Part model, mm, in its own coordinate system. Round coordinates to 2 decimals unless told otherwise and drop trailing zeros. Write each loop counter-clockwise with the first axis right and the second up, starting at its lowest first coordinate (ties: lowest second). Pieces come first, ordered by that corner, then holes. Notation, with made-up numbers: (5, 89) -> (57, 89) arc R25 ccw to (57, 124) -> close; hole circle Ø9 at (32, 1). An arc over 180 degrees is marked (long way). Return JSON: item names as keys, results as strings. Group by question number.
```python
from build123d import *

# Parameters (mm, degrees)
SKETCH1_W            = 44
SKETCH1_H            = 45.6
BOSS_EXTRUDE1_DEPTH  = 18
FILLET1_R            = 3
M4_CLEARANCE_HOLE1_D = 4.5


with BuildPart() as part:
    # Sketch1 → Boss-Extrude1 (new body)
    with BuildSketch(Plane(origin=(0, 0, 0), x_dir=(1, 0, 0), z_dir=(0, 1, 0))):
        Rectangle(SKETCH1_W, SKETCH1_H)
    extrude(amount=BOSS_EXTRUDE1_DEPTH)

    # Fillet1
    fillet1_edges = [part.edges().sort_by_distance(p)[0] for p in [
        (22, 9, 22.8),
        (-22, 9, 22.8),
        (-22, 9, -22.8),
        (22, 9, -22.8),
    ]]
    fillet(fillet1_edges, radius=FILLET1_R)

    # M4 Clearance Hole1 (through all)
    with Locations(Plane(origin=(0, 18, 0), x_dir=(1, 0, 0), z_dir=(0, 1, 0))):
        with Locations((15.25, -15.25), (-15.25, 15.25), (-15.25, -15.25), (15.25, 15.25)):
            Hole(M4_CLEARANCE_HOLE1_D / 2)


solid = part.part
```
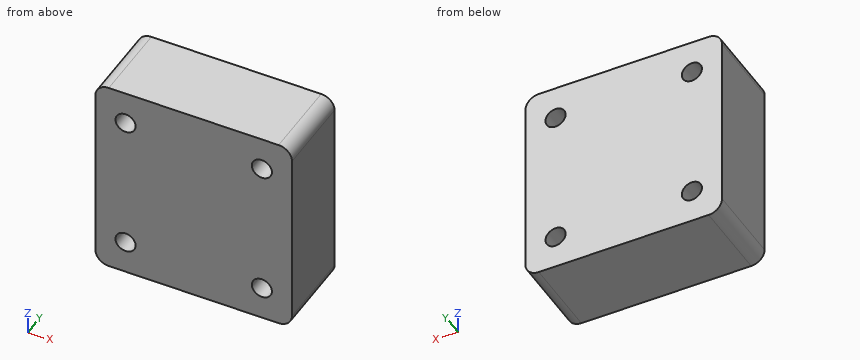
Item 1: Cut at C-C (y = 10.75). Write the cut outline in (x, z).
Item 2: Flat gauge pins, fed straight in: P1, Ø7, axis at x = -15.25, z = -15.25, coming from the +Y side; P2, Ø2.5, axis at x = 15.25, z = -15.25, coming from the -Y side. Where does each tip first touch, or does it go through?
Item 3: Wall check: L1, parallel to X at y = 4.5, z = -15.25; L2, parallel to Z at x = -15.25, y = 10.5; L3, parallel to Z at x = 17, y = 12.75. Give the ranges that are in metal, low to high.
Item 4: Cut at B-B (z = -15.25). Write the cut outline in (x, y).
Item 5: Cut at A-A (x = -15.25). Write the cut outline in (y, z).
Checks:
{
 "1": {"outline": "(-22, -19.8) arc R3 ccw to (-19, -22.8) -> (19, -22.8) arc R3 ccw to (22, -19.8) -> (22, 19.8) arc R3 ccw to (19, 22.8) -> (-19, 22.8) arc R3 ccw to (-22, 19.8) -> close; hole circle Ø4.5 at (-15.25, -15.25); hole circle Ø4.5 at (-15.25, 15.25); hole circle Ø4.5 at (15.25, -15.25); hole circle Ø4.5 at (15.25, 15.25)"},
 "2": {"P1": "stops at y = 18", "P2": "passes through"},
 "3": {"L1": "x = -22 to -17.5, -13 to 13, 17.5 to 22", "L2": "z = -22.8 to -17.5, -13 to 13, 17.5 to 22.8", "L3": "z = -22.8 to -16.66, -13.84 to 13.84, 16.66 to 22.8"},
 "4": {"outline": "(-22, 0) -> (-17.5, 0) -> (-17.5, 18) -> (-22, 18) -> close; (-13, 0) -> (13, 0) -> (13, 18) -> (-13, 18) -> close; (17.5, 0) -> (22, 0) -> (22, 18) -> (17.5, 18) -> close"},
 "5": {"outline": "(0, -22.8) -> (18, -22.8) -> (18, -17.5) -> (0, -17.5) -> close; (0, -13) -> (18, -13) -> (18, 13) -> (0, 13) -> close; (0, 17.5) -> (18, 17.5) -> (18, 22.8) -> (0, 22.8) -> close"}
}
